```python
from build123d import *

# Parameters (mm, degrees)
F0_R     = 30.467504
F1_DEPTH = 187.6
F2_W     = 13.727636
F2_H     = 54.504935
F2_W_2   = 30.864643
F2_H_2   = 20.4884
F2_W_3   = 38.292515
F2_H_3   = 10.689599
F2_W_4   = 11.208073
F2_H_4   = 33.850385
F3_DEPTH = 25
F4_R     = 2.716617
F4_R_2   = 2.765864
F4_R_3   = 3.189043
F4_R_4   = 3.014963
F5_DEPTH = 159


with BuildPart() as f1:
    # F0 (on Top) → F1 (new body)
    with BuildSketch(Plane.XY):
        Circle(F0_R)
    extrude(amount=-F1_DEPTH)

    # F2 (on Top) → F3 (join)
    with BuildSketch(Plane.XY):
        with Locations((6.863818, 27.252467)):
            Rectangle(F2_W, F2_H)
        with Locations((-40.128017, -1.170069)):
            Rectangle(F2_W_2, F2_H_2)
        with Locations((32.873894, -16.759068)):
            Rectangle(F2_W_3, F2_H_3)
        with Locations((-5.604036, -41.142927)):
            Rectangle(F2_W_4, F2_H_4)
    extrude(amount=F3_DEPTH)

    # F4 (on face) → F5 (join)
    with BuildSketch(Plane(origin=(0, 0, -187.6), x_dir=(1, 0, 0), z_dir=(0, 0, -1))):
        with Locations((-4.650002, 20.7)):
            Circle(F4_R)
        with Locations((20.55, 11.100001)):
            Circle(F4_R_2)
        with Locations((7.050002, -17.7)):
            Circle(F4_R_3)
        with Locations((-19.950002, 0)):
            Circle(F4_R_4)
    extrude(amount=F5_DEPTH)


solid = f1.part
```
Here's how the part is built. I have some questions about the finished solid (model axes, mm). A direction names the side the tool comes from. Give positions to 0.01 mm unless a question says otherwise; leave off trailing zeros. Order: outer loops, then holes, each group sorted by start corner. A loop starts at its lowest first (then second) coordinate and runs counter-clockwise, first axis right, second up. Notation, with made-up numbers: M 26.25,53.5 L 44.25,53.5 A24 ccw 44.25,77.5 Z; hole C 42.5,-38.75 d6. An arc over 180 degrees is marked long. Use a Markdown table: item, result. Add a question column.
1. Suppose I cut it at B-B (x = 39). List the corners of the cut face in (y, z) for me, and give its area (3 significant figures).
2. For pin 1 Ø1.5 at (x, z) = (-32, -112.5) entering from +Y; pin 2 Ø8.5 at (x, y) = (37, -14.5) entering from -Z; pin 3 Ø3 at (x, z) = (-11.5, -166.5) entering from +Y; pin 4 Ø3 at (y, z) = (-21.5, -273.5) entering from -X, each with a flat end and sliding along its axis, tell me the tip position at first contact or that it passes through.
3. Suppose I cut it at C-C (z = -88). List the corners of the cut face in (x, y) for me (1 decimal).
4. If we mould it in two halves opening along X, with no side actions, what happens to faces 5 (the flat face through (-40, -11.414, 12)), 6 (the flat face through (-24.696, -1, 12)), 7 (the flat face through (13.728, 27, 12))? For each: +X half, -X half, draft (parallel to the pull), parting line (faces both ways), or undercut.
5. On a 3-axis mill with a long thin cutter (end or side, diameter ignored), from which of +Z, -Z, +X, -X, +Y, -Y can I reach the whole of each face in a straight line? I mean faces 1 (the flat face through (33, -22.104, 12)), 2 (the flat face through (33, -11.414, 12)), 3 (the cylindrical face through (9.996, 18.921, -265.987)), 4 (the flat face through (7, 0, 12)). Say none if no direction works.
6. I need wall thicknesses on probe 1 along Y at (x, z) = (43.5, 2); probe 2 along X at (y, z) = (-0.5, -125); probe 3 along Z at (x, y) = (-3.5, 17). Which ranges of each line are inside material? Lowest first, please. Write a range as from..to.
7. Suppose I cut it at D-D (y = -51). List the corners of the cut face in (x, z) for me, and give its area (3 significant figures).
8. Suppose I cut it at A-A (z = -281). List the corners of the cut face in (x, y) for me, and give its area (3 significant figures).
Results list:
| question | item | result |
|---|---|---|
| 1 | outline | M -22.1,0 L -11.41,0 L -11.41,25 L -22.1,25 Z |
| 1 | area | 267 mm² |
| 2 | pin 1 | passes through |
| 2 | pin 2 | stops at z = 0 |
| 2 | pin 3 | stops at y = 28.78 |
| 2 | pin 4 | stops at x = -7.37 |
| 3 | outline | C 0,0 d60.9 |
| 4 | face 5 | draft |
| 4 | face 6 | undercut |
| 4 | face 7 | +X half |
| 5 | face 1 | +Z, +X, -X, -Y |
| 5 | face 2 | +Z, +X, +Y |
| 5 | face 3 | -Z |
| 5 | face 4 | +Z, +X, -Y |
| 6 | probe 1 | y = -22.1..-11.41 |
| 6 | probe 2 | x = -30.46..30.46 |
| 6 | probe 3 | z = -187.6..0 |
| 7 | outline | M -11.21,0 L 0,0 L 0,25 L -11.21,25 Z |
| 7 | area | 280 mm² |
| 8 | outline | C -19.95,0 d6.03; C -4.65,-20.7 d5.43; C 7.05,17.7 d6.38; C 20.55,-11.1 d5.53 |
| 8 | area | 108 mm² |
